from build123d import *

# Parameters (mm, degrees)
BOSS_EXTRUDE1_DEPTH     = 40
SKETCH2_W               = 10
SKETCH2_H               = 30
SKETCH2_H_2             = 10
CUT_EXTRUDE1_DEPTH      = 40
CUT_EXTRUDE1_DEPTH_BACK = 40


with BuildPart() as part:
    # Sketch1 → Boss-Extrude1 (new body)
    with BuildSketch(Plane.XY):
        with BuildLine():
            Line((-20, 0), (-20, -20))
            Line((-20, -20), (20, -20))
            Line((20, -20), (20, 0))
            ThreePointArc((20, 0), (0, 20), (-20, 0))
        make_face()
    extrude(amount=BOSS_EXTRUDE1_DEPTH)

    # Sketch2 → Cut-Extrude1 (cut, two sides)
    with BuildSketch(Plane(origin=(0, 0, 0), x_dir=(0, 0, -1), z_dir=(1, 0, 0))) as cut_extrude1_sk:
        with Locations((-5, -5)):
            Rectangle(SKETCH2_W, SKETCH2_H)
        with Locations((-25, 15)):
            Rectangle(SKETCH2_W, SKETCH2_H_2)
    extrude(amount=CUT_EXTRUDE1_DEPTH, mode=Mode.SUBTRACT)
    extrude(cut_extrude1_sk.sketch, amount=-CUT_EXTRUDE1_DEPTH_BACK, mode=Mode.SUBTRACT)


solid = part.part
Source: CAD feature listing. Evaluate the final solid. Frame: model axes, mm. A direction names the side the tool comes from. Give positions to 0.01 mm unless a question says otherwise; leave off trailing zeros. Write each loop counter-clockwise with the first axis right and the second up, starting at its lowest first coordinate (ties: lowest second). Pieces come first, ordered by that corner, then holes. Notation, with made-up numbers: M -3,-4.75 L 11,-4.75 A29 ccw 11,22.25 Z; hole C 73,9 d3. An arc over 180 degrees is marked long. Return JSON: item names as keys, results as strings. Group by question number.
1) Pin query (flat end, axial travel): P1, Ø8, axis at x = 4, z = 3.5, coming from the -Y side; P2, Ø10, axis at x = 15.5, z = 9.5, coming from the +Y side; P3, Ø3, axis at x = -8.5, z = 4.5, coming from the +Y side (3 decimals); P4, Ø3, axis at x = 0.5, y = 13.5, coming from the -Z side. Return the tip coordinate at first contact, or that it passes through.
2) Cut plane B-B, the plane z = 11. Output: boundary loops of the cut face in (x, y).
3) Material intervals for line 1 along Z through (x, y) = (9.5, 14.5); line 2 along Y through (x, z) = (11, 25.5); line 3 along Z through (x, y) = (-10.5, 1.5), sorted ascending. Write a range as [from, to].
4) Cut plane C-C, the plane y = -7. Output: boundary loops of the cut face in (x, z), plus the area to 3 significant figures.
5) Pull-direction query (Z, two-part tool) for faces 1 (the face through (0, 0, 40)), 2 (the face through (0, -20, 25)), 3 (the face through (0, 10, 25)); classes: pulls with the +Z half, pulls with the -Z half, needs draft (parallel to the pull), parting line crosses it, or undercut.
6) Cut plane D-D, the plane x = 13. Output: boundary loops of the cut face in (y, z).
7) Set-up query: faces 4 (the face through (0, 14, 20)), 5 (the face through (0, 10, 5)), 6 (the face through (-20, -10, 25)). Return all of +Z, -Z, +X, -X, +Y, -Y with unobstructed straight access to the full face (end or side cutting, diameter ignored); none if empty.
8) Cut plane A-A, the plane x = 0. Output: boundary loops of the cut face in (y, z).
Recorded:
{
 "1": {"P1": "stops at y = 10", "P2": "stops at y = 17.02", "P3": "stops at y = 18.735", "P4": "stops at z = 0"},
 "2": {"outline": "M -20,-20 L 20,-20 L 20,0 A20 ccw -20,0 Z"},
 "3": {"line 1": "z = [0, 20], [30, 40]", "line 2": "y = [-20, 10]", "line 3": "z = [10, 40]"},
 "4": {"outline": "M -20,10 L 20,10 L 20,40 L -20,40 Z", "area": "1,200 mm²"},
 "5": {"face 1": "pulls with the +Z half", "face 2": "needs draft", "face 3": "undercut"},
 "6": {"outline": "M -20,10 L 10,10 L 10,0 L 15.2,0 L 15.2,20 L 10,20 L 10,30 L 15.2,30 L 15.2,40 L -20,40 Z"},
 "7": {"face 4": "+X, -X, +Y", "face 5": "-Z, +X, -X, -Y", "face 6": "+Z, -Z, -X, +Y, -Y"},
 "8": {"outline": "M -20,10 L 10,10 L 10,0 L 20,0 L 20,20 L 10,20 L 10,30 L 20,30 L 20,40 L -20,40 Z"}
}
